Autodesk Inventor part; units mm, degrees
ref_plane "YZ Plane" through (0, 0, 0) normal (1, 0, 0) x (0, 1, 0)
ref_plane "XZ Plane" through (0, 0, 0) normal (0, 1, 0) x (-1, 0, 0)
ref_plane "XY Plane" through (0, 0, 0) normal (0, 0, 1) x (1, 0, 0)
sketch "Sketch1" plane through (0, 0, 0) normal (0, 0, 1) x (1, 0, 0)
  line L0 (20, -90.5) -> (20, 90.5)
  line L1 (-20, 90.5) -> (-20, -90.5)
  line L2 (-20, -90.5) -> (20, 90.5) construction
  line L3 (20, -90.5) -> (-20, 90.5) construction
  line L4 (-2.5, 90.5) -> (-2.5, 93.5)
  line L5 (-2.5, 93.5) -> (-12.5, 93.5)
  line L6 (-12.5, 93.5) -> (-12.5, 90.5)
  line L7 (12.5, 90.5) -> (12.5, 93.5)
  line L8 (12.5, 93.5) -> (2.5, 93.5)
  line L9 (2.5, 93.5) -> (2.5, 90.5)
  line L10 (12.5, 90.5) -> (20, 90.5)
  line L11 (-2.5, 90.5) -> (2.5, 90.5)
  line L12 (-20, 90.5) -> (-12.5, 90.5)
  line L13 (-20, -90.5) -> (-12.5, -90.5)
  line L14 (-12.5, -90.5) -> (-12.5, -93.5)
  line L15 (-12.5, -93.5) -> (-2.5, -93.5)
  line L16 (-2.5, -93.5) -> (-2.5, -90.5)
  line L17 (-2.5, -90.5) -> (2.5, -90.5)
  line L18 (2.5, -90.5) -> (2.5, -93.5)
  line L19 (2.5, -93.5) -> (12.5, -93.5)
  line L20 (12.5, -93.5) -> (12.5, -90.5)
  line L21 (12.5, -90.5) -> (20, -90.5)
  point P0 (0, 0)
  dimension "d0" = 40
  dimension "d1" = 181
  dimension "d2" = 10
  dimension "d3" = 3
  dimension "d4" = 7.5
  dimension "d5" = 10
  dimension "d6" = 3
  dimension "d7" = 5
  dimension "d8" = 7.5
  dimension "d9" = 3
  dimension "d10" = 10
  dimension "d11" = 5
  dimension "d12" = 3
  dimension "d13" = 10
  dimension "d14" = 3
  dimension "d15" = 12.462
  dimension "d16" = 90
  dimension "d17" = 0
extrude "Extrusion1" add sketch "Sketch1" along normal blind 3
sketch "Sketch2" plane through (0, 0, 3) normal (0, 0, 1) x (1, 0, 0)
  line L0 (-7.5, -70.5) -> (7.5, -70.5)
  line L1 (7.5, -70.5) -> (7.5, -75.5)
  line L2 (7.5, -75.5) -> (-7.5, -75.5)
  line L3 (-7.5, -75.5) -> (-7.5, -70.5)
  line L4 (-7.5, -70.5) -> (7.5, -75.5) construction
  line L5 (7.5, -70.5) -> (-7.5, -75.5) construction
  line L6 (-2.5, -90.5) -> (2.5, -90.5)
  line L7 (-20, 90.5) -> (-20, -90.5)
  point P0 (0, 0)
  point P1 (0, -73)
  dimension "d20" = 15
  dimension "d21" = 5
  dimension "d22" = 15
  dimension "d23" = 12.5
extrude "Extrusion2" cut sketch "Sketch2" against normal blind 10
equation "\"BendRadius\" = Thickness"
equation "\"BendReliefWidth\" = Thickness"
equation "\"BendReliefDepth\" = 0.5 * Thickness"
equation "\"CornerReliefSize\" = 4 * Thickness"
equation "\"MinimumRemnant\" = 2 * Thickness"
equation "\"TransitionRadius\" = BendRadius"
equation "\"JacobiRadiusSize\" = BendRadius"
equation "\"GapSize\" = Thickness"
properties part number "4 binnen dikke cover plaat"
Geometry: final body of the model. Coordinates: model frame, mm. A direction names the side the tool comes from. Give positions to 0.01 mm unless a question says otherwise; leave off trailing zeros. Loops run counter-clockwise (first coordinate to the right, second up) from the corner with the lowest first, then second, coordinate; pieces in that order, holes last. Notation, with made-up numbers: (30, 67.25) -> (88, 67.25) arc R10 cw to (88, 71.25) -> close; hole circle Ø10 at (65.25, -1). An arc over 180 degrees is marked (long way). Return JSON: item names as keys, results as strings.
Item 1: Mould query, pull axis X, two halves, no side actions, for faces 1 (the flat face through (0, 1, 3)), 2 (the flat face through (-2.5, 92, 1)), 3 (the flat face through (12.5, 92, 1)), 4 (the flat face through (0, -75.5, 2)). Classes: released by +X, released by -X, zero draft, split by the parting line, or undercut.
Filled in:
{"face 1": "zero draft", "face 2": "undercut", "face 3": "released by +X", "face 4": "undercut"}
Item 2: Pin query (flat end, axial travel): P1, Ø0.9, axis at y = 92, z = 2, coming from the +X side; P2, Ø0.9, axis at y = 92, z = 2, coming from the -X side; P3, Ø1.5, axis at x = 17, z = 1, coming from the -Y side. Return the tip coordinate at first contact, or that it passes through.
Filled in:
{"P1": "x = 12.5", "P2": "x = -12.5", "P3": "y = -90.5"}
Item 3: Access query for faces 5 (the flat face through (2.5, -92, 1)), 6 (the flat face through (-12.5, -92, 1)), 7 (the flat face through (16, -90.5, 1)), 8 (the flat face through (16, 90.5, 1)), 9 (the flat face through (-12.5, 92, 1)). Directions: +Z, -Z, +X, -X, +Y, -Y. A direction counts if a zero-diameter tool reaches every point of the face in a straight line with its end or side. Return the directions, or none.
Filled in:
{"face 5": "+Z, -Z, -Y", "face 6": "+Z, -Z, -X, -Y", "face 7": "+Z, -Z, +X, -Y", "face 8": "+Z, -Z, +X, +Y", "face 9": "+Z, -Z, -X, +Y"}
Item 4: Line query: line 1 (X direction, y = -72.5, z = 0.35); line 2 (Y direction, x = 0.5, z = 0.5); line 3 (Y direction, x = -4, z = 2.7). Output: solid intervals per line, ascending.
Filled in:
{"line 1": "-20 to -7.5, 7.5 to 20", "line 2": "-90.5 to -75.5, -70.5 to 90.5", "line 3": "-93.5 to -75.5, -70.5 to 93.5"}
Item 5: Section A-A, the plane x = 0. Output: boundary loops of the cut face in (y, z), plus the area to 3 significant figures.
Filled in:
{"outline": "(-90.5, 0) -> (-75.5, 0) -> (-75.5, 3) -> (-90.5, 3) -> close; (-70.5, 0) -> (90.5, 0) -> (90.5, 3) -> (-70.5, 3) -> close", "area": "528 mm^2"}
Item 6: Section B-B, the plane z = 0.5. Output: boundary loops of the cut face in (x, y).
Filled in:
{"outline": "(-20, -90.5) -> (-12.5, -90.5) -> (-12.5, -93.5) -> (-2.5, -93.5) -> (-2.5, -90.5) -> (2.5, -90.5) -> (2.5, -93.5) -> (12.5, -93.5) -> (12.5, -90.5) -> (20, -90.5) -> (20, 90.5) -> (12.5, 90.5) -> (12.5, 93.5) -> (2.5, 93.5) -> (2.5, 90.5) -> (-2.5, 90.5) -> (-2.5, 93.5) -> (-12.5, 93.5) -> (-12.5, 90.5) -> (-20, 90.5) -> close; hole (-7.5, -75.5) -> (7.5, -75.5) -> (7.5, -70.5) -> (-7.5, -70.5) -> close"}
